from build123d import *

# Parameters (mm, degrees)
EXTRUDE_THIN1_DEPTH = 449.2625
CUT_EXTRUDE1_START  = -8.5
CUT_EXTRUDE1_DEPTH  = 9.5
LPATTERN1_COUNT     = 18
LPATTERN1_PITCH     = 25
FILLET1_R           = 0.5
SKETCH5_W           = 14.543721181
SKETCH5_H           = 38.348187902
CUT_EXTRUDE2_DEPTH  = 93.6625


with BuildPart() as part:
    # Sketch3 → Extrude-Thin1 (new body)
    with BuildSketch(Plane.XY):
        Polygon((-6.5, 17.5), (-6.5, 13.5), (0, 13.5), (0, -13.5), (-6.5, -13.5), (-6.5, -17.5), (-7.5, -17.5), (-7.5, -12.5), (-1, -12.5), (-1, 12.5), (-7.5, 12.5), (-7.5, 17.5), align=None)
    extrude(amount=EXTRUDE_THIN1_DEPTH)

    # Sketch4 → Cut-Extrude1 (cut)
    with BuildSketch(Plane(origin=(0, 0, 0), x_dir=(0, 0, -1), z_dir=(1, 0, 0)).offset(CUT_EXTRUDE1_START)):
        with BuildLine():
            Line((-6.65, -3.15), (-18.35, -3.15))
            ThreePointArc((-18.35, -3.15), (-21.5, 0), (-18.35, 3.15))
            Line((-18.35, 3.15), (-6.65, 3.15))
            ThreePointArc((-6.65, 3.15), (-3.5, 0), (-6.65, -3.15))
        make_face()
    cut_extrude1 = extrude(amount=CUT_EXTRUDE1_DEPTH, mode=Mode.SUBTRACT)

    # LPattern1: Cut-Extrude1 ×18
    with Locations(*[(0, 0, i * LPATTERN1_PITCH) for i in range(1, LPATTERN1_COUNT)]):
        add(cut_extrude1, mode=Mode.SUBTRACT)

    # Fillet1
    fillet1_edges = [part.edges().sort_by_distance(p)[0] for p in [
        (-6.5, 13.5, 224.63125),
        (0, 13.5, 224.63125),
        (0, -13.5, 224.63125),
        (-6.5, -13.5, 224.63125),
        (-7.5, -12.5, 224.63125),
        (-1, -12.5, 224.63125),
        (-1, 12.5, 224.63125),
        (-7.5, 12.5, 224.63125),
    ]]
    fillet(fillet1_edges, radius=FILLET1_R)

    # Sketch5 → Cut-Extrude2 (cut)
    with BuildSketch(Plane.XY.offset(449.2625)):
        with Locations((-3.04454966, -0.3205253)):
            Rectangle(SKETCH5_W, SKETCH5_H)
    extrude(amount=-CUT_EXTRUDE2_DEPTH, mode=Mode.SUBTRACT)


solid = part.part
CAD build for the part. Positions are in the model's coordinates, mm. A direction names the side the tool comes from. Give positions to 0.01 mm unless a question says otherwise; leave off trailing zeros. Write each loop counter-clockwise with the first axis right and the second up, starting at its lowest first coordinate (ties: lowest second). Pieces come first, ordered by that corner, then holes. Notation, with made-up numbers: (7.25, 18.5) - (17.25, 18.5) arc R21 cw to (17.25, 40.5) - close; hole circle Ø3 at (41.25, -14.75). An arc over 180 degrees is marked (long way). Put each result on its own line as item: value.
(1) Saw through at A-A (x = -4.75). List the corners of the cut face in (y, z).
Working result:
outline: (-13.5, 0) - (-12.5, 0) - (-12.5, 355.6) - (-13.5, 355.6) - close; (12.5, 0) - (13.5, 0) - (13.5, 355.6) - (12.5, 355.6) - close
(2) Saw through at D-D (y = 9). List the corners of the cut face in (x, z), then the cut area to 3 significant figures.
Working result:
outline: (-1, 0) - (0, 0) - (0, 355.6) - (-1, 355.6) - close
area: 356 mm^2
(3) Saw through at C-C (z = 250.5). List the corners of the cut face in (x, y).
Working result:
outline: (-7.5, -17.5) - (-6.5, -17.5) - (-6.5, -14) arc R0.5 cw to (-6, -13.5) - (-0.5, -13.5) arc R0.5 ccw to (0, -13) - (0, 13) arc R0.5 ccw to (-0.5, 13.5) - (-6, 13.5) arc R0.5 cw to (-6.5, 14) - (-6.5, 17.5) - (-7.5, 17.5) - (-7.5, 13) arc R0.5 ccw to (-7, 12.5) - (-1.5, 12.5) arc R0.5 cw to (-1, 12) - (-1, -12) arc R0.5 cw to (-1.5, -12.5) - (-7, -12.5) arc R0.5 ccw to (-7.5, -13) - close
(4) Pull direction Y, two halves, no side cores. Call faces 1 (the flat face through (-3, -13.5, 175)), 2 (the flat face through (-4, 12.5, 175)), 3 (the flat face through (-0.7, -1.2, 0)): released by +Y, released by -Y, zero draft, split by the parting line, or undercut.
Working result:
face 1: released by -Y
face 2: undercut
face 3: zero draft
(5) Wall check: L1, parallel to Y at x = -4.75, z = 287; L2, parallel to Y at x = -6.75, z = 241; L3, parallel to X at y = -4.5, z = 16.5. Give the ranges that are in metal, low to high.
Working result:
L1: -13.5 to -12.5, 12.5 to 13.5
L2: -17.5 to -12.5, 12.5 to 17.5
L3: -1 to 0
(6) Saw through at B-B (z = 64.5). List the corners of the cut face in (x, y), then the cut area to 3 significant figures.
Working result:
outline: (-7.5, -17.5) - (-6.5, -17.5) - (-6.5, -14) arc R0.5 cw to (-6, -13.5) - (-0.5, -13.5) arc R0.5 ccw to (0, -13) - (0, -3.15) - (-1, -3.15) - (-1, -12) arc R0.5 cw to (-1.5, -12.5) - (-7, -12.5) arc R0.5 ccw to (-7.5, -13) - close; (-7.5, 13) arc R0.5 ccw to (-7, 12.5) - (-1.5, 12.5) arc R0.5 cw to (-1, 12) - (-1, 3.15) - (0, 3.15) - (0, 13) arc R0.5 ccw to (-0.5, 13.5) - (-6, 13.5) arc R0.5 cw to (-6.5, 14) - (-6.5, 17.5) - (-7.5, 17.5) - close
area: 41.7 mm^2
(7) Tool access for faces 4 (the flat face through (-1, 0, 175)), 5 (the flat face through (-3, -13, 355.6)), 6 (the flat face through (-3, 13.5, 175)): list every direction of +Z, -Z, +X, -X, +Y, -Y with a clear straight run to the whole face (end or side of a thin tool).
Working result:
face 4: +Z, -Z, -X
face 5: +Z, +X, -X, +Y, -Y
face 6: +Z, -Z, +X, +Y
(8) Drop flat-ended pins along their axis: pin 1 Ø3 at (y, z) = (16, 245.5) entering from +X; pin 2 Ø2 at (x, y) = (-1.5, 1.5) entering from +Z; pin 3 Ø1.1 at (x, z) = (-0.5, 186.5) entering from -Y; pin 4 Ø4.5 at (x, z) = (-4.5, 125) entering from +Y. Give the stop position or say it passes through.
Working result:
pin 1: x = -6.5
pin 2: z = 354.57
pin 3: y = -13.5
pin 4: y = 17.5
